```python
from build123d import *

# Parameters (mm, degrees)
ESQUISSE1_W             = 10
ESQUISSE1_H             = 30
ESQUISSE1_R             = 1.75
BOSS_EXTRU_1_DEPTH      = 20
ESQUISSE2_W             = 10
ESQUISSE2_H             = 30
BOSS_EXTRU_2_DEPTH      = 10
ESQUISSE3_W             = 10
ESQUISSE3_H             = 27
BOSS_EXTRU_3_DEPTH      = 30
ESQUISSE4_R             = 1.75
ENL_V_MAT_EXTRU_1_DEPTH = 15


with BuildPart() as part:
    # Esquisse1 → Boss.-Extru.1 (new body)
    with BuildSketch(Plane.XY):
        with Locations((5, 15)):
            Rectangle(ESQUISSE1_W, ESQUISSE1_H)
        with Locations((5, 5)):
            Circle(ESQUISSE1_R, mode=Mode.SUBTRACT)
        with Locations((5, 15)):
            Circle(ESQUISSE1_R, mode=Mode.SUBTRACT)
        with Locations((5, 25)):
            Circle(ESQUISSE1_R, mode=Mode.SUBTRACT)
    extrude(amount=BOSS_EXTRU_1_DEPTH)

    # Esquisse2 → Boss.-Extru.2 (add)
    with BuildSketch(Plane.XY.offset(20)):
        with Locations((5, 15)):
            Rectangle(ESQUISSE2_W, ESQUISSE2_H)
    extrude(amount=BOSS_EXTRU_2_DEPTH)

    # Esquisse3 → Boss.-Extru.3 (add)
    with BuildSketch(Plane.XY.offset(30)):
        with Locations((5, 16.5)):
            Rectangle(ESQUISSE3_W, ESQUISSE3_H)
    extrude(amount=BOSS_EXTRU_3_DEPTH)

    # Esquisse4 → Enlèv. mat.-Extru.1 (cut)
    with BuildSketch(Plane(origin=(0, 3, 0), x_dir=(-1, 0, 0), z_dir=(0, -1, 0))):
        with Locations(Location((-5, -55, 0), (0, 0, 180))):
            Circle(ESQUISSE4_R)
        with Locations(Location((-5, -45, 0), (0, 0, 180))):
            Circle(ESQUISSE4_R)
        with Locations(Location((-5, -35, 0), (0, 0, 180))):
            Circle(ESQUISSE4_R)
    extrude(amount=-ENL_V_MAT_EXTRU_1_DEPTH, mode=Mode.SUBTRACT)


solid = part.part
```
Check sheet for the modelled part. Datum: model origin and axes. Units: mm. A direction names the side the tool comes from. Give positions to 0.01 mm unless a question says otherwise; leave off trailing zeros. Order: outer loops, then holes, each group sorted by start corner. A loop starts at its lowest first (then second) coordinate and runs counter-clockwise, first axis right, second up. Notation, with made-up numbers: M 74,-31.75 L 107,-31.75 A22 ccw 107,-6.75 Z; hole C -27.75,2 d11. An arc over 180 degrees is marked long. Answer in a Markdown table with one row per item. Add a question column.
Q1. Sectioned sample at A-A, the plane y = 11.5. Record the boundary of the cut face in (x, z), and give its area (3 significant figures).
Q2. Gauge pin test, flat ends, axial feed: pin 1 Ø3 at (x, y) = (5, 15) entering from -Z; pin 2 Ø3 at (x, z) = (6, 35.5) entering from -Y; pin 3 Ø2 at (x, z) = (5, 45) entering from -Y. Record the tip position at first contact, or that the pin passes through.
Q3. Sectioned sample at D-D, the plane z = 18. Record the boundary of the cut face in (x, y).
Q4. Release check for a two-part mould opening along X. For faces 1 (the flat face through (5, 18, 45)), 2 (the flat face through (5, 0, 15)), 3 (the flat face through (10, 15, 30)) record: released by +X, released by -X, zero draft, split by the parting line, or undercut.
Q5. Access from +Z, -Z, +X, -X, +Y, -Y to the whole of each face (thin tool, end or side, straight path). Record for faces 4 (the cylindrical face through (4.62, 10.4, 43.29)), 5 (the cylindrical face through (3.61, 3.94, 9.86)), 6 (the flat face through (0, 15, 30)), 7 (the flat face through (7, 15, 0)), 8 (the flat face through (7, 3, 45)).
Q6. Thickness scan on L1, parallel to Y at x = 5, z = 5; L2, parallel to Z at x = 5, y = 8.75; L3, parallel to Z at x = 6.5, y = 10. Record the ranges inside material, lowest first.
Q7. Sectioned sample at B-B, the plane z = 45. Record the boundary of the cut face in (x, y), and give its area (4 significant figures).
Q8. Sectioned sample at C-C, the plane y = 25. Record the boundary of the cut face in (x, z), and give its area (3 significant figures).
Verdict:
| question | item | result |
|---|---|---|
| 1 | outline | M 0,0 L 10,0 L 10,60 L 0,60 Z; hole C 5,35 d3.5; hole C 5,45 d3.5; hole C 5,55 d3.5 |
| 1 | area | 571 mm² |
| 2 | pin 1 | z = 20 |
| 2 | pin 2 | y = 3 |
| 2 | pin 3 | y = 18 |
| 3 | outline | M 0,0 L 10,0 L 10,30 L 0,30 Z; hole C 5,5 d3.5; hole C 5,15 d3.5; hole C 5,25 d3.5 |
| 4 | face 1 | undercut |
| 4 | face 2 | zero draft |
| 4 | face 3 | released by +X |
| 5 | face 4 | -Y |
| 5 | face 5 | -Z |
| 5 | face 6 | +Z, -Z, -X, +Y, -Y |
| 5 | face 7 | -Z, +X, -X, +Y, -Y |
| 5 | face 8 | +Z, +X, -X, -Y |
| 6 | L1 | 0 to 3.25, 6.75 to 13.25, 16.75 to 23.25, 26.75 to 30 |
| 6 | L2 | 0 to 33.25, 36.75 to 43.25, 46.75 to 53.25, 56.75 to 60 |
| 6 | L3 | 0 to 34.1, 35.9 to 44.1, 45.9 to 54.1, 55.9 to 60 |
| 7 | outline | M 0,3 L 3.25,3 L 3.25,18 L 6.75,18 L 6.75,3 L 10,3 L 10,30 L 0,30 Z |
| 7 | area | 217.5 mm² |
| 8 | outline | M 0,0 L 3.25,0 L 3.25,20 L 6.75,20 L 6.75,0 L 10,0 L 10,60 L 0,60 Z |
| 8 | area | 530 mm² |
